Read the model definition and answer for the solid it produces. Units are mm, in the model's axes. Face numbers are marked on the shaded views. Coordinates: 2 decimals unless noted, no trailing zeros. Loops run counter-clockwise (first coordinate to the right, second up) from the corner with the lowest first, then second, coordinate; pieces in that order, holes last. Notation, with made-up numbers: M 34,37 L 91,37 A15 ccw 91,65 Z; hole C 81,-25.5 d4. An arc over 180 degrees is marked long. One line per item, written item: value. Start each with the question number.
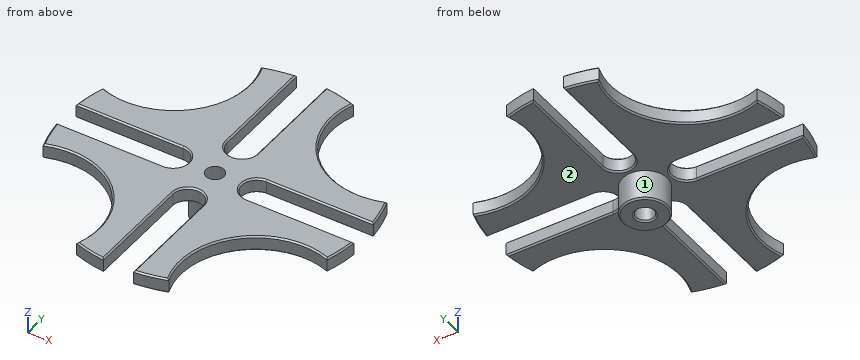
```python
from build123d import *

# Parameters (mm, degrees)
SKETCH1_R                = 50
SKETCH1_R_2              = 3
BOSS_EXTRUDE1_DEPTH      = 5
SKETCH2_R                = 25
CUT_EXTRUDE1_DEPTH       = 71.887234394
CHAMFER1_SIZE            = 0.5
BOSS_EXTRUDE3_DEPTH      = 10
BOSS_EXTRUDE3_DEPTH_BACK = 5
SKETCH4_R                = 7.5
SKETCH4_R_2              = 3
CHAMFER2_SIZE            = 0.5


with BuildPart() as part:
    # Sketch1 → Boss-Extrude1 (new body)
    with BuildSketch(Plane.XY):
        Circle(SKETCH1_R)
        Circle(SKETCH1_R_2, mode=Mode.SUBTRACT)
    extrude(amount=BOSS_EXTRUDE1_DEPTH)

    # Sketch2 → Cut-Extrude1 (cut, through all)
    with BuildSketch(Plane.XY.offset(5)):
        with Locations((38.890872965, 38.890872965)):
            Circle(SKETCH2_R)
        with Locations((38.890872965, -38.890872965)):
            Circle(SKETCH2_R)
        with Locations((-38.890872965, -38.890872965)):
            Circle(SKETCH2_R)
        with Locations((-38.890872965, 38.890872965)):
            Circle(SKETCH2_R)
        with BuildLine():
            Line((-5, 14), (-5, 86))
            ThreePointArc((-5, 86), (0, 91), (5, 86))
            Line((5, 86), (5, 14))
            ThreePointArc((5, 14), (0, 9), (-5, 14))
        make_face()
        with BuildLine():
            Line((14, 5), (86, 5))
            ThreePointArc((86, 5), (91, 0), (86, -5))
            Line((86, -5), (14, -5))
            ThreePointArc((14, -5), (9, 0), (14, 5))
        make_face()
        with BuildLine():
            Line((5, -14), (5, -86))
            ThreePointArc((5, -86), (0, -91), (-5, -86))
            Line((-5, -86), (-5, -14))
            ThreePointArc((-5, -14), (0, -9), (5, -14))
        make_face()
        with BuildLine():
            Line((-14, -5), (-86, -5))
            ThreePointArc((-86, -5), (-91, 0), (-86, 5))
            Line((-86, 5), (-14, 5))
            ThreePointArc((-14, 5), (-9, 0), (-14, -5))
        make_face()
    extrude(amount=-CUT_EXTRUDE1_DEPTH, mode=Mode.SUBTRACT)

    # Chamfer1
    chamfer1_edges = [part.edges().sort_by_distance(p)[0] for p in [
        (-10.27898673, 48.932018473, 0),
        (-5, 31.874685928, 0),
        (5, 31.874685928, 0),
        (5, 31.874685928, 5),
        (-5, 31.874685928, 5),
        (0, 9, 5),
        (0, 9, 0),
        (-48.932018473, 10.27898673, 5),
        (-48.932018473, -10.27898673, 5),
        (-10.27898673, -48.932018473, 5),
        (10.27898673, -48.932018473, 5),
        (48.932018473, -10.27898673, 5),
        (48.932018473, 10.27898673, 5),
        (10.27898673, 48.932018473, 5),
        (-48.932018473, 10.27898673, 0),
        (-48.932018473, -10.27898673, 0),
        (-10.27898673, -48.932018473, 0),
        (10.27898673, -48.932018473, 0),
        (48.932018473, -10.27898673, 0),
        (48.932018473, 10.27898673, 0),
        (10.27898673, 48.932018473, 0),
        (-3, 0, 0),
        (-3, 0, 5),
        (-31.874685928, -5, 0),
        (-31.874685928, 5, 0),
        (-31.874685928, 5, 5),
        (-31.874685928, -5, 5),
        (-9, 0, 5),
        (-9, 0, 0),
        (21.213203436, -21.213203436, 0),
        (21.213203436, -21.213203436, 5),
        (-21.213203436, -21.213203436, 0),
        (-21.213203436, -21.213203436, 5),
        (-21.213203436, 21.213203436, 0),
        (-21.213203436, 21.213203436, 5),
        (5, -31.874685928, 0),
        (-5, -31.874685928, 0),
        (-5, -31.874685928, 5),
        (5, -31.874685928, 5),
        (0, -9, 5),
        (0, -9, 0),
        (31.874685928, 5, 0),
        (31.874685928, -5, 0),
        (31.874685928, -5, 5),
        (31.874685928, 5, 5),
        (9, 0, 5),
        (9, 0, 0),
        (21.213203436, 21.213203436, 0),
        (21.213203436, 21.213203436, 5),
        (-10.27898673, 48.932018473, 5),
    ]]
    chamfer(chamfer1_edges, length=CHAMFER1_SIZE)

    # Sketch4 → Boss-Extrude3 (add, two sides: drawn at the far end of the back side and taken through both)
    with BuildSketch(Plane(origin=(0, 0, 0), x_dir=(-1, 0, 0), z_dir=(0, 0, -1)).offset(-BOSS_EXTRUDE3_DEPTH_BACK)):
        Circle(SKETCH4_R)
        Circle(SKETCH4_R_2, mode=Mode.SUBTRACT)
    extrude(amount=BOSS_EXTRUDE3_DEPTH + BOSS_EXTRUDE3_DEPTH_BACK)

    # Chamfer2
    chamfer2_edges = [part.edges().sort_by_distance(p)[0] for p in [
        (3, 0, -10),
        (7.5, 0, -10),
    ]]
    chamfer(chamfer2_edges, length=CHAMFER2_SIZE)


solid = part.part
```
1) Section B-B (z = -8) is taken. Determine the outline of the cut face in (x, y), then the cut area to 3 significant figures.
2) For a pull along X with two mould halves and no side action, classify the marked faces 1 and 2 as released by +X, released by -X, zero draft, split by the parting line, or undercut.
3) Section A-A (z = 2.25) is taken. Determine the outline of the cut face in (x, y), then the cut area to 3 significant figures.
4) Consider line 1 along Y through (x, z) = (0, 0.75); line 2 along Y through (x, z) = (0, -4); line 3 along Z through (x, y) = (20, -10). Determine where each line is inside the solid, lowest interval first.
5) Flat-ended cylindrical pins translate along their axes: pin 1 (4.5 mm diameter, centred on y = 23, z = 2, fed in from -X); pin 2 (3 mm diameter, centred on y = -23, z = 2.5, fed in from -X); pin 3 (3 mm diameter, centred on x = 31, z = 1.5, fed in from -Y); pin 4 (8 mm diameter, centred on x = 0, y = 0, fed in from +Z). Find the tip coordinate at first contact, or state that the pin passes through.
Results found:
1. outline: C 0,0 d15; hole C 0,0 d6
1. area: 148 mm²
2. face 1: split by the parting line
2. face 2: zero draft
3. outline: M -49.75,-5 A50 ccw -47.56,-15.44 A25 cw -15.44,-47.56 A50 ccw -5,-49.75 L -5,-14 A5 cw 5,-14 L 5,-49.75 A50 ccw 15.44,-47.56 A25 cw 47.56,-15.44 A50 ccw 49.75,-5 L 14,-5 A5 cw 14,5 L 49.75,5 A50 ccw 47.56,15.44 A25 cw 15.44,47.56 A50 ccw 5,49.75 L 5,14 A5 cw -5,14 L -5,49.75 A50 ccw -15.44,47.56 A25 cw -47.56,15.44 A50 ccw -49.75,5 L -14,5 A5 cw -14,-5 Z; hole C 0,0 d6
3. area: 3,670 mm²
4. line 1: y = -9 to -3, 3 to 9
4. line 2: y = -7.5 to -3, 3 to 7.5
4. line 3: z = 0 to 5
5. pin 1: stops at x = -21.69
5. pin 2: stops at x = -20.93
5. pin 3: stops at y = -15.72
5. pin 4: stops at z = 5
